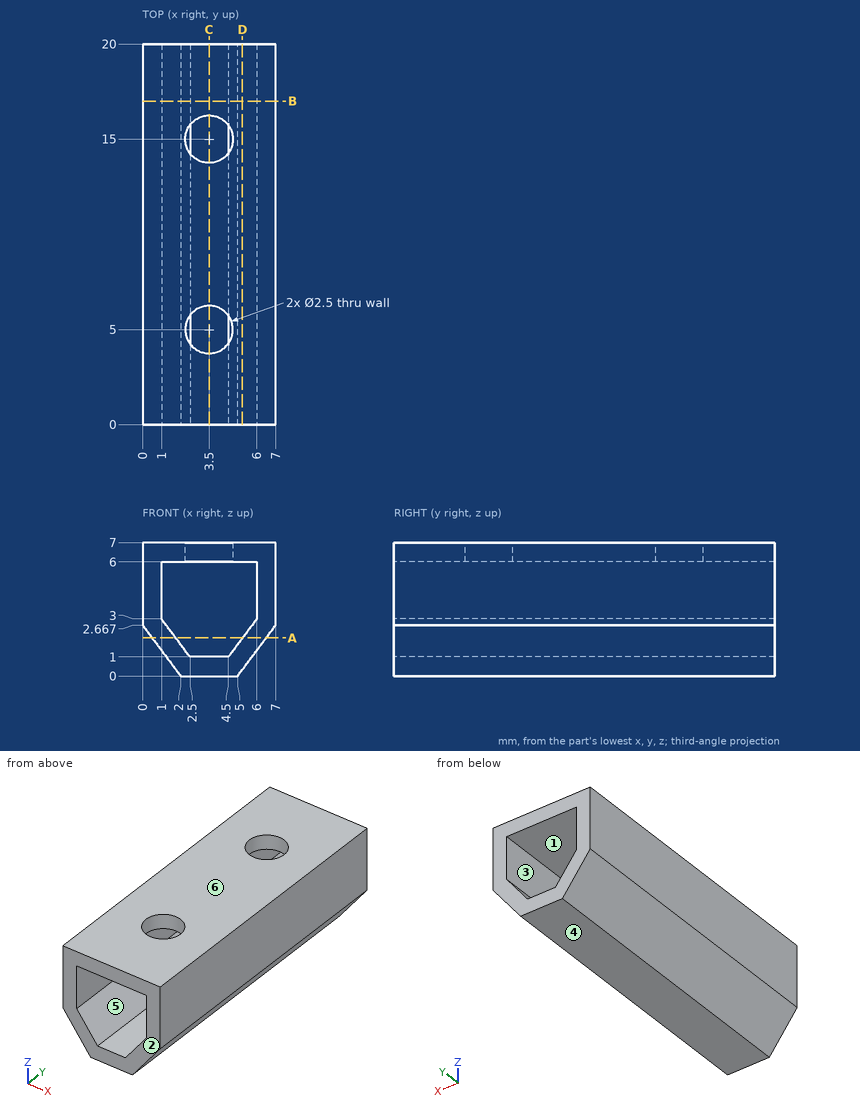
Design review of the part shown in the three views and the two pictorial views. Dimensions are in mm from the part's minimum x, y and z. A direction names the side the tool comes from. Round coordinates to 2 decimals unless told otherwise and drop trailing zeros. Loops run counter-clockwise (first coordinate to the right, second up) from the corner with the lowest first, then second, coordinate; pieces in that order, holes last. Notation, with made-up numbers: (20, 72.25) - (50, 72.25) arc R18 cw to (50, 88.25) - close; hole circle Ø7 at (-25, -26.75). An arc over 180 degrees is marked (long way). Answer as CSV lines item,"result".
(1) Consider section B-B on y = 17. Give the boundary of the cut face in (x, z).
Checked values:
outline,"(0, 2.67) - (2, 0) - (5, 0) - (7, 2.67) - (7, 7) - (0, 7) - close; hole (1, 3) - (2.5, 1) - (4.5, 1) - (6, 3) - (6, 6) - (1, 6) - close"
(2) Mouldability with a two-part tool opening along Z and no side actions: class the marked faces 1, 2, 3 and 4 as +Z half, -Z half, draft (parallel to the pull), parting line (faces both ways), or undercut.
Checked values:
face 1,"undercut"
face 2,"draft"
face 3,"undercut"
face 4,"-Z half"
(3) Insertion check: P1, Ø1.5, axis at x = 4.5, z = 4, coming from the -Y side. The pin has a flat end and moves straight along its axis. Give the tip position at first contact, or say it passes through.
Checked values:
P1,"passes through"
(4) Consider section A-A on z = 2. Give the boundary of the cut face in (x, y).
Checked values:
outline,"(0.5, 0) - (1.75, 0) - (1.75, 20) - (0.5, 20) - close; (5.25, 0) - (6.5, 0) - (6.5, 20) - (5.25, 20) - close"
(5) Consider section C-C on x = 3.5. Give the boundary of the cut face in (y, z).
Checked values:
outline,"(0, 0) - (20, 0) - (20, 1) - (0, 1) - close; (0, 6) - (3.75, 6) - (3.75, 7) - (0, 7) - close; (6.25, 6) - (13.75, 6) - (13.75, 7) - (6.25, 7) - close; (16.25, 6) - (20, 6) - (20, 7) - (16.25, 7) - close"
(6) Consider section D-D on x = 5.25. Give the boundary of the cut face in (y, z).
Checked values:
outline,"(0, 0.33) - (20, 0.33) - (20, 2) - (0, 2) - close; (0, 6) - (20, 6) - (20, 7) - (0, 7) - close"
(7) Tool access review of the marked faces 5 and 6: name each direction out of +Z, -Z, +X, -X, +Y, -Y from which nothing blocks a thin tool from reaching the whole face with its end or side.
Checked values:
face 5,"+Y, -Y"
face 6,"+Z, +X, -X, +Y, -Y"
(8) Wall thickness on line 1 (Y direction, x = 3.5, z = 6.45); line 2 (X direction, y = 15, z = 6.35); line 3 (Z direction, x = 2.75, y = 8.75): over which ranges is each line inside the solid? List them lowest first.
Checked values:
line 1,"y = 0 to 3.75, 6.25 to 13.75, 16.25 to 20"
line 2,"x = 0 to 2.25, 4.75 to 7"
line 3,"z = 0 to 1, 6 to 7"
